from build123d import *

# Parameters (mm, degrees)
SKETCH1_W           = 37.465
SKETCH1_H           = 24.13
BOSS_EXTRUDE1_DEPTH = 4.445
CUT_EXTRUDE2_DEPTH  = 2.54
FILLET1_R           = 5.08
CUT_EXTRUDE4_DEPTH  = 2.54
SKETCH4_R           = 1.27
CUT_EXTRUDE5_DEPTH  = 2.54
SKETCH5_R           = 1.905
SKETCH5_R_2         = 1.27
CUT_EXTRUDE6_DEPTH  = 0.635
CUT_EXTRUDE7_DEPTH  = 2.54


with BuildPart() as part:
    # Sketch1 → Boss-Extrude1 (new body)
    with BuildSketch(Plane.XY):
        with Locations((18.7325, 12.065)):
            Rectangle(SKETCH1_W, SKETCH1_H)
    extrude(amount=BOSS_EXTRUDE1_DEPTH)

    # Sketch2 → Cut-Extrude2 (cut)
    # profile 1 of 4: a face of its own
    with BuildSketch(Plane.XY.offset(4.445)):
        with BuildLine():
            Line((35.59175, 5.7785), (35.59175, 12.065))
            Line((35.59175, 12.065), (35.59175, 18.3515))
            ThreePointArc((35.59175, 18.3515), (34.135361545, 21.710109865), (30.681521372, 22.9235))
            Line((30.681521372, 22.9235), (18.7325, 22.9235))
            Line((18.7325, 22.9235), (6.107021372, 22.9235))
            ThreePointArc((6.107021372, 22.9235), (3.090639267, 21.470453234), (1.87325, 18.3515))
            Line((1.87325, 18.3515), (1.87325, 12.065))
            Line((1.87325, 12.065), (1.87325, 5.7785))
            ThreePointArc((1.87325, 5.7785), (3.212357796, 2.545607796), (6.44525, 1.2065))
            Line((6.44525, 1.2065), (18.7325, 1.2065))
            Line((18.7325, 1.2065), (31.01975, 1.2065))
            ThreePointArc((31.01975, 1.2065), (34.252642204, 2.545607796), (35.59175, 5.7785))
        make_face()
        with BuildLine():
            ThreePointArc((7.493, 3.175), (4.439712919, 4.439712919), (3.175, 7.493))
            Line((3.175, 7.493), (3.175, 16.637))
            ThreePointArc((3.175, 16.637), (4.317872951, 19.576666289), (7.154771372, 20.955))
            Line((7.154771372, 20.955), (7.493, 20.955))
            Line((7.493, 20.955), (29.633771372, 20.955))
            ThreePointArc((29.633771372, 20.955), (32.908147923, 19.81638289), (34.29, 16.637))
            Line((34.29, 16.637), (34.29, 7.493))
            ThreePointArc((34.29, 7.493), (33.025287081, 4.439712919), (29.972, 3.175))
            Line((29.972, 3.175), (7.493, 3.175))
        make_face(mode=Mode.SUBTRACT)
    # profile 2 of 4: a face of its own
    with BuildSketch(Plane.XY.offset(4.445)):
        with BuildLine():
            ThreePointArc((3.175, 16.637), (4.439712919, 19.690287081), (7.493, 20.955))
            Line((7.493, 20.955), (29.972, 20.955))
            ThreePointArc((29.972, 20.955), (33.025287081, 19.690287081), (34.29, 16.637))
            Line((34.29, 16.637), (34.29, 7.493))
            ThreePointArc((34.29, 7.493), (33.025287081, 4.439712919), (29.972, 3.175))
            Line((29.972, 3.175), (7.493, 3.175))
            ThreePointArc((7.493, 3.175), (4.439712919, 4.439712919), (3.175, 7.493))
            Line((3.175, 7.493), (3.175, 16.637))
        make_face()
    # profile 3 of 4: a face of its own
    with BuildSketch(Plane.XY.offset(4.445)):
        with BuildLine():
            ThreePointArc((7.154771372, 20.955), (4.317872951, 19.576666289), (3.175, 16.637))
            ThreePointArc((3.175, 16.637), (4.439712919, 19.690287081), (7.493, 20.955))
            Line((7.493, 20.955), (7.154771372, 20.955))
        make_face()
    # profile 4 of 4: a face of its own
    with BuildSketch(Plane.XY.offset(4.445)):
        with BuildLine():
            ThreePointArc((34.29, 16.637), (32.908147923, 19.81638289), (29.633771372, 20.955))
            Line((29.633771372, 20.955), (29.972, 20.955))
            ThreePointArc((29.972, 20.955), (33.025287081, 19.690287081), (34.29, 16.637))
        make_face()
    extrude(amount=-CUT_EXTRUDE2_DEPTH, mode=Mode.SUBTRACT)

    # Fillet1
    fillet1_edges = [part.edges().sort_by_distance(p)[0] for p in [
        (0, 24.13, 2.2225),
        (37.465, 24.13, 2.2225),
        (37.465, 0, 2.2225),
        (0, 0, 2.2225),
    ]]
    fillet(fillet1_edges, radius=FILLET1_R)

    # Sketch3 → Cut-Extrude4 (cut)
    with BuildSketch(Plane.XY.offset(1.905)):
        with BuildLine():
            Line((7.350869654, 16.158973759), (18.677995313, 16.158973759))
            ThreePointArc((18.677995313, 16.158973759), (21.522821275, 14.644991178), (22.463869654, 11.5628481))
            Line((22.463869654, 11.5628481), (22.463869654, 7.801099417))
            ThreePointArc((22.463869654, 7.801099417), (21.522821275, 4.718956339), (18.677995313, 3.204973759))
            Line((18.677995313, 3.204973759), (7.350869654, 3.204973759))
            ThreePointArc((7.350869654, 3.204973759), (4.387385134, 4.432489239), (3.159869654, 7.395973759))
            Line((3.159869654, 7.395973759), (3.159869654, 11.967973759))
            ThreePointArc((3.159869654, 11.967973759), (4.387385134, 14.931458278), (7.350869654, 16.158973759))
        make_face()
    extrude(amount=-CUT_EXTRUDE4_DEPTH, mode=Mode.SUBTRACT)

    # Sketch4 → Cut-Extrude5 (cut)
    with BuildSketch(Plane.XY.offset(1.905)):
        with Locations((27.511650569, 9.68988988)):
            Circle(SKETCH4_R)
    extrude(amount=-CUT_EXTRUDE5_DEPTH, mode=Mode.SUBTRACT)

    # Sketch5 → Cut-Extrude6 (cut)
    with BuildSketch(Plane.XY.offset(1.905)):
        with Locations((27.511650569, 9.68988988)):
            Circle(SKETCH5_R)
        with Locations((27.511650569, 9.68988988)):
            Circle(SKETCH5_R_2, mode=Mode.SUBTRACT)
    extrude(amount=-CUT_EXTRUDE6_DEPTH, mode=Mode.SUBTRACT)

    # Sketch6 → Cut-Extrude7 (cut)
    with BuildSketch(Plane.XY.offset(4.445)):
        with BuildLine():
            Line((1.542829573, 18.47723), (1.542829573, 5.65277))
            ThreePointArc((1.542829573, 5.65277), (2.908719525, 2.355219952), (6.206269573, 0.98933))
            Line((6.206269573, 0.98933), (31.272259573, 0.98933))
            ThreePointArc((31.272259573, 0.98933), (34.56980962, 2.355219952), (35.935699573, 5.65277))
            Line((35.935699573, 5.65277), (35.935699573, 18.47723))
            ThreePointArc((35.935699573, 18.47723), (34.450183348, 21.903012063), (30.927266372, 23.14067))
            Line((30.927266372, 23.14067), (5.861276372, 23.14067))
            ThreePointArc((5.861276372, 23.14067), (2.784566625, 21.658562299), (1.542829573, 18.47723))
        make_face()
        with BuildLine():
            Line((6.44525, 1.2065), (31.01975, 1.2065))
            ThreePointArc((31.01975, 1.2065), (34.252642204, 2.545607796), (35.59175, 5.7785))
            Line((35.59175, 5.7785), (35.59175, 18.3515))
            ThreePointArc((35.59175, 18.3515), (34.135361545, 21.710109865), (30.681521372, 22.9235))
            Line((30.681521372, 22.9235), (6.107021372, 22.9235))
            ThreePointArc((6.107021372, 22.9235), (3.090639267, 21.470453234), (1.87325, 18.3515))
            Line((1.87325, 18.3515), (1.87325, 5.7785))
            ThreePointArc((1.87325, 5.7785), (3.212357796, 2.545607796), (6.44525, 1.2065))
        make_face(mode=Mode.SUBTRACT)
    extrude(amount=-CUT_EXTRUDE7_DEPTH, mode=Mode.SUBTRACT)


solid = part.part
The model under review builds one solid part; all positions refer to its coordinate system, in mm. A direction names the side the tool comes from. Give positions to 0.01 mm unless a question says otherwise; leave off trailing zeros. Loops run counter-clockwise (first coordinate to the right, second up) from the corner with the lowest first, then second, coordinate; pieces in that order, holes last. Notation, with made-up numbers: (53.25, 15.25) -> (62.25, 15.25) arc R25 cw to (62.25, 33.25) -> close; hole circle Ø3 at (19.25, 11). An arc over 180 degrees is marked (long way). Answer as a JSON object with one key per item and string values. Group by question number.
Q1. Draft analysis for pull direction X (two halves, no side actions). For faces 1 (the flat face through (35.936, 12, 3)), 2 (the flat face through (23, 12, 0)), 3 (the flat face through (37.465, 12, 2)), state which applies: pulls with the +X half, pulls with the -X half, needs draft (parallel to the pull), parting line crosses it, or undercut.
Q2. Wall thickness on line 1 along Y through (x, z) = (27.5, 1.8); line 2 along Y through (x, z) = (13.5, 0.55); line 3 along X through (y, z) = (12, 3.7) (3 decimals): over which ranges is each line inside the solid? List them lowest first.
Q3. Take a section at B-B (z = 3.4). Write out the cut boundary in (x, y) (3 decimals), plus the area to 3 significant figures.
Q4. Take a section at A-A (x = 8). Write out the cut boundary in (y, z) (3 decimals), plus the area to 3 significant figures.
Q5. Tool access review of faces 4 (the cylindrical face through (21.493, 14.681, 0.966)), 5 (the cylindrical face through (34.533, 2.319, 3.193)), 6 (the flat face through (17.3, 0.5, 4.445)): name each direction out of +Z, -Z, +X, -X, +Y, -Y from which nothing blocks a thin tool from reaching the whole face with its end or side.
Q6. Insertion check: pin 1 (6 mm diameter, centred on x = 32, y = 14, fed in from -Z); pin 2 (6.5 mm diameter, centred on x = 24.5, y = 11, fed in from +Z) (3 decimals); pin 3 (1.9 mm diameter, centred on x = 27, y = 9, fed in from +Z); pin 4 (1.5 mm diameter, centred on x = 27.51, y = 9.69, fed in from +Z). Each pin has a flat end and moves straight along its axis. Give the tip position at first contact, or say it passes through.
Q7. Take a section at C-C (y = 16.75). Write out the cut boundary in (x, z) (3 decimals), plus the area to 3 significant figures.
Q8. Take a section at D-D (z = 0.6). Write out the cut boundary in (x, y) (3 decimals), plus the area to 3 significant figures.
Answer below:
{
 "1": {"face 1": "undercut", "face 2": "needs draft", "face 3": "pulls with the +X half"},
 "2": {"line 1": "y = 0 to 7.78, 11.59 to 24.13", "line 2": "y = 0 to 3.2, 16.16 to 24.13", "line 3": "x = 0 to 1.543, 35.936 to 37.465"},
 "3": {"outline": "(0, 5.08) arc R5.08 ccw to (5.08, 0) -> (32.385, 0) arc R5.08 ccw to (37.465, 5.08) -> (37.465, 19.05) arc R5.08 ccw to (32.385, 24.13) -> (5.08, 24.13) arc R5.08 ccw to (0, 19.05) -> close; hole (1.543, 5.653) arc R4.663 ccw to (6.206, 0.989) -> (31.272, 0.989) arc R4.663 ccw to (35.936, 5.653) -> (35.936, 18.477) arc R4.663 ccw to (30.927, 23.141) -> (5.861, 23.141) arc R4.663 ccw to (1.543, 18.477) -> close", "area": "139 mm2"},
 "4": {"outline": "(0, 0) -> (3.205, 0) -> (3.205, 1.905) -> (0.989, 1.905) -> (0.989, 4.445) -> (0, 4.445) -> close; (16.159, 0) -> (24.13, 0) -> (24.13, 4.445) -> (23.141, 4.445) -> (23.141, 1.905) -> (16.159, 1.905) -> close", "area": "26.3 mm2"},
 "5": {"face 4": "+Z, -Z", "face 5": "+Z", "face 6": "+Z, +X, -X, +Y, -Y"},
 "6": {"pin 1": "stops at z = 0", "pin 2": "stops at z = 1.905", "pin 3": "stops at z = 1.27", "pin 4": "passes through"},
 "7": {"outline": "(0, 0) -> (37.465, 0) -> (37.465, 4.445) -> (35.936, 4.445) -> (35.936, 1.905) -> (1.543, 1.905) -> (1.543, 4.445) -> (0, 4.445) -> close", "area": "79.2 mm2"},
 "8": {"outline": "(0, 5.08) arc R5.08 ccw to (5.08, 0) -> (32.385, 0) arc R5.08 ccw to (37.465, 5.08) -> (37.465, 19.05) arc R5.08 ccw to (32.385, 24.13) -> (5.08, 24.13) arc R5.08 ccw to (0, 19.05) -> close; hole (3.16, 7.396) arc R4.191 ccw to (7.351, 3.205) -> (18.678, 3.205) arc R4.211 ccw to (22.464, 7.801) -> (22.464, 11.563) arc R4.211 ccw to (18.678, 16.159) -> (7.351, 16.159) arc R4.191 ccw to (3.16, 11.968) -> close; hole circle Ø2.54 at (27.512, 9.69)", "area": "642 mm2"}
}
